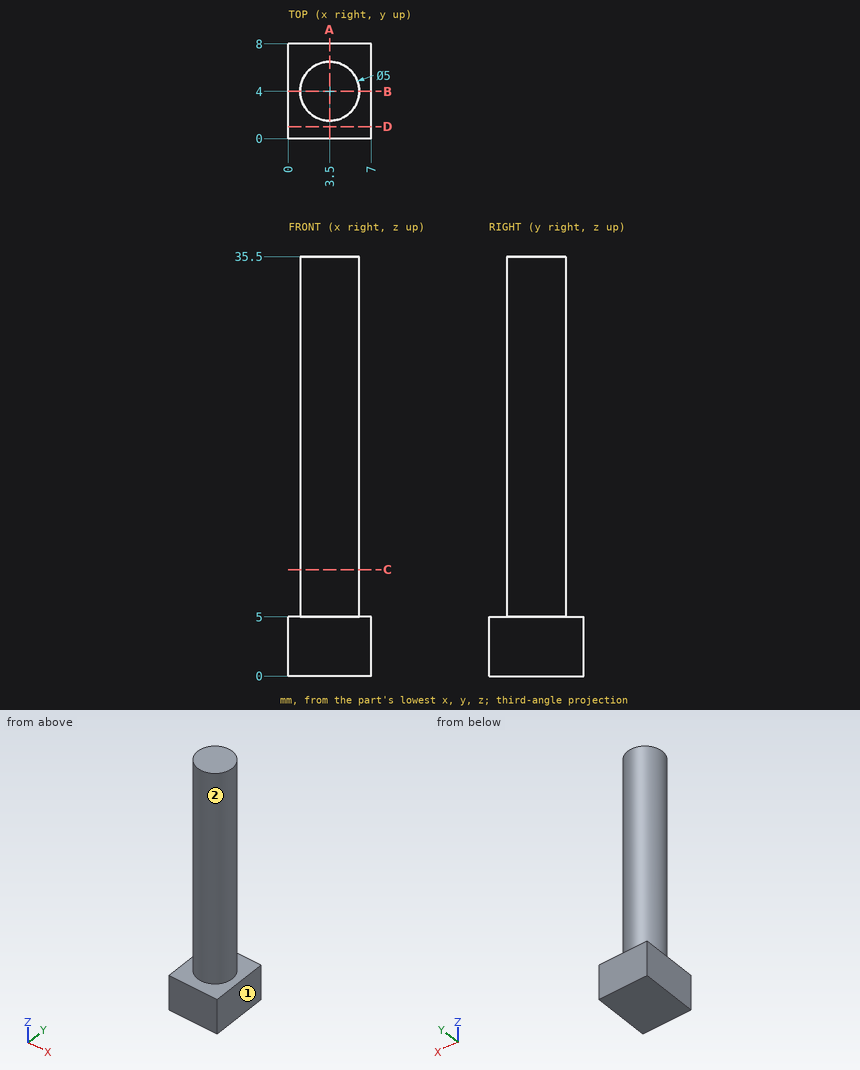
Geometry check sheet. Reference: drawing and pictorial views, mm from the part's lowest x, y, z. A direction names the side the tool comes from. Coordinates: 2 decimals unless noted, no trailing zeros. Write each loop counter-clockwise with the first axis right and the second up, starting at its lowest first coordinate (ties: lowest second). Pieces come first, ordered by that corner, then holes. Notation, with made-up numbers: M 86,-1 L 131,-1 A24 cw 131,17 Z; hole C -7,54 d7. An arc over 180 degrees is marked long. One line per question, with ' | ' between items.
1) Access from +Z, -Z, +X, -X, +Y, -Y to the whole of each face (thin tool, end or side, straight path). Record for the marked faces 1 and 2.
Solutions:
face 1: +Z, -Z, +X, +Y, -Y | face 2: +Z
2) Sectioned sample at B-B on y = 4. Record the cut outline in (x, z), then the cut area to 4 significant figures.
Solutions:
outline: M 0,0 L 7,0 L 7,5 L 6,5 L 6,35.5 L 1,35.5 L 1,5 L 0,5 Z | area: 187.5 mm^2
3) Sectioned sample at D-D on y = 1. Record the cut outline in (x, z).
Solutions:
outline: M 0,0 L 7,0 L 7,5 L 0,5 Z
4) Material ranges on L1, parallel to Z at x = 4, y = 7; L2, parallel to Y at x = 3.75, z = 12.5; L3, parallel to X at y = 3.5, z = 30, recorded low to high.
Solutions:
L1: 0 to 5 | L2: 1.51 to 6.49 | L3: 1.05 to 5.95
5) Sectioned sample at C-C on z = 9. Record the cut outline in (x, y).
Solutions:
outline: C 3.5,4 d5
6) Sectioned sample at A-A on x = 3.5. Record the cut outline in (y, z).
Solutions:
outline: M 0,0 L 8,0 L 8,5 L 6.5,5 L 6.5,35.5 L 1.5,35.5 L 1.5,5 L 0,5 Z
7) Depth check by flat-ended pin: pin 1 Ø4 at (y, z) = (5.5, 28) entering from -X; pin 2 Ø1.5 at (x, z) = (3, 7) entering from +Y; pin 3 Ø1.5 at (y, z) = (3, 17.5) entering from +X; pin 4 Ø3 at (x, y) = (6, 2) entering from -Z. Enter the tip coordinate at first touch or a pass-through.
Solutions:
pin 1: x = 1 | pin 2: y = 6.5 | pin 3: x = 5.99 | pin 4: z = 0
